Geometry: final body of the model. Coordinates: model frame, mm. Give positions to 0.01 mm unless a question says otherwise; leave off trailing zeros. Write each loop counter-clockwise with the first axis right and the second up, starting at its lowest first coordinate (ties: lowest second). Pieces come first, ordered by that corner, then holes. Notation, with made-up numbers: (53, 41.5) -> (95, 41.5) arc R21 cw to (95, 78.5) -> close; hole circle Ø2 at (49, 37.25). An arc over 180 degrees is marked (long way). Answer as a JSON object with one key per item and string values. Group by question number.
(1) Contact query for a flat-ended pin moving along its axis: pin 1 Ø2.5 at (x, y) = (0.5, 0.5) entering from -Z. Output: stop coordinate, or through.
(2) Section query A-A on z = 125.5. Output: boundary loops of the cut face in (x, y).
(3) Material intervals for probe 1 along Y at (x, z) = (0, 7); probe 2 along Y at (x, z) = (0, 3), sorted ascending.
from build123d import *

# Parameters (mm, degrees)
ESQUISSE1_R               = 2.5
BOSS_EXTRU_1_DEPTH        = 340
ESQUISSE2_OUTSIDE_W       = 75.014
ESQUISSE2_OUTSIDE_H       = 75.014
ESQUISSE2_OUTSIDE_R       = 2
ENL_V_MAT_EXTRU_1_DEPTH   = 4.2
TROU_TARAUD_M3X0_51_D     = 2.5
TROU_TARAUD_M3X0_51_DEPTH = 8.5
TROU_TARAUD_M3X0_51_TIP   = 0.751075774


with BuildPart() as part:
    # Esquisse1 → Boss.-Extru.1 (new body)
    with BuildSketch(Plane.XY):
        Circle(ESQUISSE1_R)
    extrude(amount=BOSS_EXTRU_1_DEPTH)

    # Esquisse2 outside → Enlèv. mat.-Extru.1 (cut)
    with BuildSketch(Plane(origin=(0, 0, 0), x_dir=(-1, 0, 0), z_dir=(0, 0, -1))):
        Rectangle(ESQUISSE2_OUTSIDE_W, ESQUISSE2_OUTSIDE_H)
        Circle(ESQUISSE2_OUTSIDE_R, mode=Mode.SUBTRACT)
    extrude(amount=-ENL_V_MAT_EXTRU_1_DEPTH, mode=Mode.SUBTRACT)

    # Trou taraudé M3x0.51
    with Locations(Plane(origin=(0, 0, 0), x_dir=(-1, 0, 0), z_dir=(0, 0, -1))):
        with Locations((0, 0)):
            Hole(TROU_TARAUD_M3X0_51_D / 2, depth=TROU_TARAUD_M3X0_51_DEPTH)
            with Locations((0, 0, -(TROU_TARAUD_M3X0_51_DEPTH + TROU_TARAUD_M3X0_51_TIP / 2))):  # 118° drill point
                Cone(0, TROU_TARAUD_M3X0_51_D / 2, TROU_TARAUD_M3X0_51_TIP, mode=Mode.SUBTRACT)


solid = part.part
Answer list:
{
 "1": {"pin 1": "z = 0"},
 "2": {"outline": "circle Ø5 at (0, 0)"},
 "3": {"probe 1": "-2.5 to -1.25, 1.25 to 2.5", "probe 2": "-2 to -1.25, 1.25 to 2"}
}
